```python
from build123d import *

# Parameters (mm, degrees)
BOSS_EXTRUDE1_DEPTH   = 36.425
CUT_EXTRUDE1_DEPTH    = 110.090212662
CUT_EXTRUDE2_DEPTH    = 109.098783751
FILLET1_R             = 3
BOSS_EXTRUDE12_REACH  = 92.552
BOSS_EXTRUDE12_START  = -4.21
SKETCH27_W            = 1.5
SKETCH27_H            = 5
CUT_EXTRUDE9_REACH    = 101.691
SKETCH30_W            = 0.716863464
SKETCH30_H            = 2.5
SKETCH31_R            = 0.9
BOSS_EXTRUDE13_DEPTH  = 1
FILLET9_R             = 1.5
FILLET10_R            = 1.5
FILLET11_R            = 0.9
FILLET9_OF_MIRROR4_R  = 1.5
FILLET10_OF_MIRROR4_R = 1.5
FILLET11_OF_MIRROR4_R = 0.9
FILLET12_R            = 0.5


with BuildPart() as part:
    # Sketch1 → Boss-Extrude1 (new, symmetric)
    with BuildSketch(Plane.XY):
        with BuildLine():
            Line((0, 0), (-17.110884891, -59.672747116))
            ThreePointArc((-17.110884891, -59.672747116), (-22.347799076, -68.454296451), (-31.240591359, -73.5))
            Line((-31.240591359, -73.5), (-30.858426801, -74.9505))
            ThreePointArc((-30.858426801, -74.9505), (-21.298675096, -69.526368685), (-15.668992347, -60.08620315))
            Line((-15.668992347, -60.08620315), (1.441892544, -0.413456034))
            Line((1.441892544, -0.413456034), (1.560449154, 0))
            Line((1.560449154, 0), (0, 0))
        make_face()
    extrude(amount=BOSS_EXTRUDE1_DEPTH, both=True)

    # Sketch2 → Cut-Extrude1 (cut, through all)
    with BuildSketch(Plane.XY.offset(36.425)):
        with BuildLine():
            Line((-31.240591359, -73.5), (-26.943866684, -73.5))
            ThreePointArc((-26.943866684, -73.5), (-28.865857957, -74.320486174), (-30.858426801, -74.9505))
            Line((-30.858426801, -74.9505), (-31.240591359, -73.5))
        make_face()
    extrude(amount=-CUT_EXTRUDE1_DEPTH, mode=Mode.SUBTRACT)

    # Sketch3 → Cut-Extrude2 (cut, through all)
    with BuildSketch(Plane.XY.offset(36.425)):
        with BuildLine():
            Line((-26.943866684, -73.5), (-31.240591359, -73.5))
            ThreePointArc((-31.240591359, -73.5), (-29.043541661, -72.783058785), (-26.943866684, -71.817451685))
            Line((-26.943866684, -71.817451685), (-26.943866684, -73.5))
        make_face()
    extrude(amount=-CUT_EXTRUDE2_DEPTH, mode=Mode.SUBTRACT)

    # Fillet1
    fillet1_edges = [part.edges().sort_by_distance(p)[0] for p in [
        (0.780224577, 0, 36.425),
        (0.780224577, 0, -36.425),
    ]]
    fillet(fillet1_edges, radius=FILLET1_R)

    # Boss-Extrude12: up to this plane
    boss_extrude12_end = Plane(origin=(0, 0, 36.425), z_dir=(0.9612616959383179, -0.2756373558170027, 0))
    # Sketch27 → Boss-Extrude12 (add, up to the surface)
    with BuildSketch(Plane(origin=(0, 0, 0), x_dir=(0, 0, -1), z_dir=(1, 0, 0)).offset(BOSS_EXTRUDE12_START), mode=Mode.PRIVATE) as boss_extrude12_sk1:
        with Locations((-24.55, 0)):
            Rectangle(SKETCH27_W, SKETCH27_H)
    boss_extrude12_tool1 = split(extrude(boss_extrude12_sk1.sketch, amount=BOSS_EXTRUDE12_REACH, mode=Mode.PRIVATE), bisect_by=boss_extrude12_end, keep=Keep.BOTH, mode=Mode.PRIVATE)
    boss_extrude12 = boss_extrude12_tool1.solids().sort_by_distance((-4.21, 0, 24.55))[0]
    add(boss_extrude12)

    # Sketch30 → Cut-Extrude9 (cut, up to next)
    with BuildSketch(Plane.XY.offset(25.3), mode=Mode.PRIVATE) as cut_extrude9_sk1:
        with Locations((0.358431732, 1.25)):
            Rectangle(SKETCH30_W, SKETCH30_H)
    cut_extrude9_tool1 = extrude(cut_extrude9_sk1.sketch, amount=-CUT_EXTRUDE9_REACH, mode=Mode.PRIVATE) & part.part
    cut_extrude9 = cut_extrude9_tool1.solids().sort_by_distance((0.358432, 1.25, 25.3))[0]
    add(cut_extrude9, mode=Mode.SUBTRACT)

    # Sketch31 → Boss-Extrude13 (add)
    with BuildSketch(Plane.XY.offset(25.3)):
        with Locations(Location((-2.21, 1, 0), (0, 0, 180))):
            Circle(SKETCH31_R)
    boss_extrude13 = extrude(amount=BOSS_EXTRUDE13_DEPTH)

    # Fillet9
    fillet9_edges = [part.edges().sort_by_distance(p)[0] for p in [
        (-4.21, 2.5, 24.55),
    ]]
    fillet(fillet9_edges, radius=FILLET9_R)

    # Fillet10
    fillet10_edges = [part.edges().sort_by_distance(p)[0] for p in [
        (0, 2.5, 24.55),
    ]]
    fillet(fillet10_edges, radius=FILLET10_R)

    # Fillet11
    fillet11_edges = [part.edges().sort_by_distance(p)[0] for p in [
        (-1.31, 1, 26.3),
    ]]
    fillet(fillet11_edges, radius=FILLET11_R)

    # Mirror4: Boss-Extrude12, Cut-Extrude9, Boss-Extrude13 across plane
    add(boss_extrude12.mirror(Plane.XY))
    add(cut_extrude9.mirror(Plane.XY), mode=Mode.SUBTRACT)
    add(boss_extrude13.mirror(Plane.XY))

    # Fillet9 of Mirror4
    fillet9_of_mirror4_edges = [part.edges().sort_by_distance(p)[0] for p in [
        (-4.21, 2.5, -24.55),
    ]]
    fillet(fillet9_of_mirror4_edges, radius=FILLET9_OF_MIRROR4_R)

    # Fillet10 of Mirror4
    fillet10_of_mirror4_edges = [part.edges().sort_by_distance(p)[0] for p in [
        (0, 2.5, -24.55),
    ]]
    fillet(fillet10_of_mirror4_edges, radius=FILLET10_OF_MIRROR4_R)

    # Fillet11 of Mirror4
    fillet11_of_mirror4_edges = [part.edges().sort_by_distance(p)[0] for p in [
        (-1.31, 1, -26.3),
    ]]
    fillet(fillet11_of_mirror4_edges, radius=FILLET11_OF_MIRROR4_R)

    # Fillet12
    fillet12_edges = [part.edges().sort_by_distance(p)[0] for p in [
        (-7.484389675, -31.543101575, 36.425),
        (-19.877867178, -67.993869785, -36.425),
        (-19.877867178, -67.993869785, 36.425),
        (-26.943866684, -73.5, 0),
        (-26.943866684, -72.658725842, -36.425),
        (-26.943866684, -72.658725842, 36.425),
        (1.560449154, 0, 0),
        (1.302457732, -0.899723012, 35.567156991),
        (1.302457732, -0.899723012, -35.567156991),
        (-7.484389675, -31.543101575, -36.425),
    ]]
    fillet(fillet12_edges, radius=FILLET12_R)

    # Chamfer1
    # the kernel refuses this chamfer: 10, 3.5 mm, written as the material it adds along each edge
    with BuildSketch(Plane(origin=(-0.716863464, -2.5, 25.3), x_dir=(-0.26268080042718955, -0.9648827892997839, 0), z_dir=(0, 0, -1))) as chamfer1_piece_1_section:
        with BuildLine():
            Line((10.375794366, 0), (0.542683512, 3.511617253))
            Line((0.542683512, 3.511617253), (0.349706955, 3.564153413))
            ThreePointArc((0.349706955, 3.564153413), (0.270766903, 1.755965125), (-0.192976558, 0.05253616))
            Line((-0.192976558, 0.05253616), (0.00269055, -0.199981902))
            ThreePointArc((0.00269055, -0.199981902), (5.189648845, -0.130196738), (10.378484916, -0.199981902))
            Line((10.378484916, -0.199981902), (10.375794366, 0))
        make_face()
    chamfer1_piece_1 = extrude(amount=1.5, mode=Mode.PRIVATE)
    chamfer1_piece_1 = split(chamfer1_piece_1, bisect_by=Plane(origin=(-4.21, -5.808119571, 24.55), z_dir=(1, 0, 0)), keep=Keep.TOP, mode=Mode.PRIVATE)
    add(chamfer1_piece_1)
    with BuildSketch(Plane(origin=(-0.716863464, -2.5, -25.3), x_dir=(-0.26268080042718955, -0.9648827892997839, 0), z_dir=(0, 0, 1))) as chamfer1_piece_2_section:
        with BuildLine():
            Line((10.375794366, 0), (0.542683512, -3.511617253))
            Line((0.542683512, -3.511617253), (0.349706955, -3.564153413))
            ThreePointArc((0.349706955, -3.564153413), (0.270766903, -1.755965125), (-0.192976558, -0.05253616))
            Line((-0.192976558, -0.05253616), (0.00269055, 0.199981902))
            ThreePointArc((0.00269055, 0.199981902), (5.189648845, 0.130196738), (10.378484916, 0.199981902))
            Line((10.378484916, 0.199981902), (10.375794366, 0))
        make_face()
    chamfer1_piece_2 = extrude(amount=1.5, mode=Mode.PRIVATE)
    chamfer1_piece_2 = split(chamfer1_piece_2, bisect_by=Plane(origin=(-4.21, -5.808119571, -24.55), z_dir=(1, 0, 0)), keep=Keep.TOP, mode=Mode.PRIVATE)
    add(chamfer1_piece_2)


solid = part.part
```
Could you check a few things on this model? Use its own coordinates, in mm. A direction names the side the tool comes from. Coordinates: 2 decimals unless noted, no trailing zeros. One line per question, with ' | ' between items. Start each with the question number.
1. Will these pins go through, and if not, where does the flat tip stop? P1, Ø8, axis at x = -22.5, z = 18, coming from the +Y side; P2, Ø1.6, axis at y = -0.5, z = -24.5, coming from the -X side; P3, Ø10, axis at x = -11.5, z = 19, coming from the -Y side.
2. For faces 1 (the face through (-21, -67, 1)), 2 (the face through (-3, -3, -23.8)), which set-ups out of +Z, -Z, +X, -X, +Y, -Y let a thin tool reach every point of the face, with its end or its side?
3. Please list where these lines run through material, in increasing order: line 1 along X through (y, z) = (-64.5, -12.5); line 2 along X through (y, z) = (-60, -7); line 3 along Y through (x, z) = (-20.5, -9.5).
4. Thinking about a two-plate mould opening in Z: for faces 3 (the face through (-8.436, -29.419, 0.51)), 4 (the face through (-10.2, -37.7, 36.425)), 5 (the face through (-10.2, -37.7, -36.425)), 6 (the face through (-3, -3, 23.8)), which applies, pulls with the +Z half, pulls with the -Z half, needs draft (parallel to the pull), parting line crosses it, or undercut?
Return value:
1) P1: stops at y = -63.21 | P2: stops at x = -4.21 | P3: stops at y = -62.45
2) face 1: +Z, -Z, -X, +Y | face 2: -X, +Y
3) line 1: x = -19.22 to -17.49 | line 2: x = -17.21 to -15.64 | line 3: y = -68.7 to -66.38
4) face 3: undercut | face 4: pulls with the +Z half | face 5: pulls with the -Z half | face 6: undercut
